Check sheet for the modelled part. Datum: model origin and axes. Units: mm. Face numbers are marked on the shaded views. A direction names the side the tool comes from. Round coordinates to 2 decimals unless told otherwise and drop trailing zeros. Write each loop counter-clockwise with the first axis right and the second up, starting at its lowest first coordinate (ties: lowest second). Pieces come first, ordered by that corner, then holes. Notation, with made-up numbers: (70, 15) -> (124, 15) arc R21 cw to (124, 33) -> close; hole circle Ø2 at (31.25, -27.75). An arc over 180 degrees is marked (long way). One line per item, written item: value.
from build123d import *

# Parameters (mm, degrees)
HORN_PLATE_ENVELOPE_PROFILE_R           = 13
HORN_PLATE_ENVELOPE_PROFILE_R_2         = 3.05
HORN_PLATE_ENVELOPE_DEPTH               = 3
SPLINE_HUB_ENVELOPE_START               = -4
SPLINE_HUB_ENVELOPE_PROFILE_R           = 4.5
SPLINE_HUB_ENVELOPE_PROFILE_R_2         = 3.05
SPLINE_HUB_ENVELOPE_DEPTH               = 4
NOMINAL_HORN_ATTACHMENT_HOLES_START     = -50
NOMINAL_HORN_ATTACHMENT_HOLES_PROFILE_R = 1.6
NOMINAL_HORN_ATTACHMENT_HOLES_DEPTH     = 69.814887722


with BuildPart() as part:
    # Horn_plate_envelope_profile → Horn_plate_envelope (new body)
    with BuildSketch(Plane.XY):
        Circle(HORN_PLATE_ENVELOPE_PROFILE_R)
        Circle(HORN_PLATE_ENVELOPE_PROFILE_R_2, mode=Mode.SUBTRACT)
    extrude(amount=HORN_PLATE_ENVELOPE_DEPTH)

    # Spline_hub_envelope_profile → Spline_hub_envelope (add)
    with BuildSketch(Plane.XY.offset(SPLINE_HUB_ENVELOPE_START)):
        Circle(SPLINE_HUB_ENVELOPE_PROFILE_R)
        Circle(SPLINE_HUB_ENVELOPE_PROFILE_R_2, mode=Mode.SUBTRACT)
    extrude(amount=SPLINE_HUB_ENVELOPE_DEPTH)

    # Nominal_horn_attachment_holes_profile → Nominal_horn_attachment_holes (cut, through all)
    with BuildSketch(Plane.XY.offset(NOMINAL_HORN_ATTACHMENT_HOLES_START)):
        with Locations((-10, 0)):
            Circle(NOMINAL_HORN_ATTACHMENT_HOLES_PROFILE_R)
        with Locations((10, 0)):
            Circle(NOMINAL_HORN_ATTACHMENT_HOLES_PROFILE_R)
        with Locations((0, -10)):
            Circle(NOMINAL_HORN_ATTACHMENT_HOLES_PROFILE_R)
        with Locations((0, 10)):
            Circle(NOMINAL_HORN_ATTACHMENT_HOLES_PROFILE_R)
    extrude(amount=NOMINAL_HORN_ATTACHMENT_HOLES_DEPTH, mode=Mode.SUBTRACT)


solid = part.part
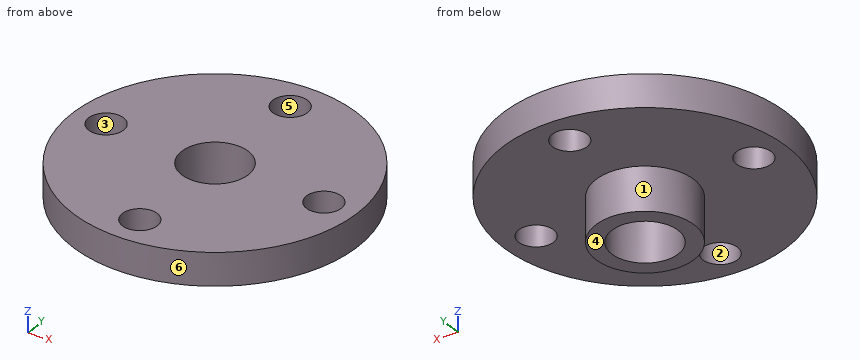
Item 1: Depth check by flat-ended pin: P1, Ø2.5, axis at x = 10, y = 0, coming from the +Z side; P2, Ø1.5, axis at x = 2.5, y = 0, coming from the +Z side; P3, Ø3, axis at x = -7, z = 1.5, coming from the -Y side; P4, Ø3.5, axis at x = -10, y = 0, coming from the -Z side. Enter the tip coordinate at first touch or a pass-through.
Answer:
P1: passes through
P2: stops at z = 3
P3: stops at y = -11.78
P4: stops at z = 0
Item 2: Tool access check on the marked faces 1 and 2. Record the directions out of +Z, -Z, +X, -X, +Y, -Y that give a thin tool (end or side, any length) a straight path to the whole face; none if there is none.
Answer:
face 1: -Z
face 2: +Z, -Z
Item 3: Sectioned sample at A-A on y = 0. Enter the section's corners in (x, z), and give its area (3 significant figures).
Answer:
outline: (-13, 0) -> (-11.6, 0) -> (-11.6, 3) -> (-13, 3) -> close; (-8.4, 0) -> (-4.5, 0) -> (-4.5, -4) -> (-3.05, -4) -> (-3.05, 3) -> (-8.4, 3) -> close; (3.05, -4) -> (4.5, -4) -> (4.5, 0) -> (8.4, 0) -> (8.4, 3) -> (3.05, 3) -> close; (11.6, 0) -> (13, 0) -> (13, 3) -> (11.6, 3) -> close
area: 52.1 mm^2
Item 4: Sectioned sample at B-B on z = 1. Enter the section's corners in (x, y), and give its area (3 significant figures).
Answer:
outline: circle Ø26 at (0, 0); hole circle Ø3.2 at (-10, 0); hole circle Ø6.1 at (0, 0); hole circle Ø3.2 at (0, -10); hole circle Ø3.2 at (0, 10); hole circle Ø3.2 at (10, 0)
area: 470 mm^2
Item 5: Sectioned sample at C-C on x = 1. Enter the section's corners in (y, z).
Answer:
outline: (-12.96, 0) -> (-11.25, 0) -> (-11.25, 3) -> (-12.96, 3) -> close; (-8.75, 0) -> (-4.39, 0) -> (-4.39, -4) -> (-2.88, -4) -> (-2.88, 3) -> (-8.75, 3) -> close; (2.88, -4) -> (4.39, -4) -> (4.39, 0) -> (8.75, 0) -> (8.75, 3) -> (2.88, 3) -> close; (11.25, 0) -> (12.96, 0) -> (12.96, 3) -> (11.25, 3) -> close
Item 6: Mould release check, pull along Y, two halves, no side actions. Record for the marked faces 3, 4, 5 and 6: pulls with the +Y half, pulls with the -Y half, needs draft (parallel to the pull), parting line crosses it, or undercut.
Answer:
face 3: undercut
face 4: needs draft
face 5: undercut
face 6: parting line crosses it
Item 7: Thickness scan on line 1 (Y direction, x = 0, z = 0.75); line 2 (Z direction, x = -5.25, y = 3); line 3 (Y direction, x = -1, z = -2). Record the ranges inside material, lowest first.
Answer:
line 1: y = -13 to -11.6, -8.4 to -3.05, 3.05 to 8.4, 11.6 to 13
line 2: z = 0 to 3
line 3: y = -4.39 to -2.88, 2.88 to 4.39
Item 8: Sectioned sample at D-D on y = 10. Enter the section's corners in (x, z).
Answer:
outline: (-8.31, 0) -> (-1.6, 0) -> (-1.6, 3) -> (-8.31, 3) -> close; (1.6, 0) -> (8.31, 0) -> (8.31, 3) -> (1.6, 3) -> close
